from build123d import *

# Parameters (mm, degrees)
SKETCH1_R           = 82.5
BOSS_EXTRUDE1_DEPTH = 28
SKETCH2_R           = 10
CUT_EXTRUDE1_DEPTH  = 120.98541578
SKETCH3_R           = 7.474835821
CUT_EXTRUDE2_DEPTH  = 19.538331
CIRPATTERN1_START   = 8.461669322
CIRPATTERN1_DEPTH   = 19.538330678


# Read off the part's stored shape, not the designer's step: CirPattern1
with BuildPart() as part:
    # Sketch1 → Boss-Extrude1 (new body)
    with BuildSketch(Plane(origin=(0, 0, 0), x_dir=(1, 0, 0), z_dir=(0, 1, 0))):
        with Locations(Location((0, 0, 0), (0, 0, 270))):
            Circle(SKETCH1_R)
    extrude(amount=BOSS_EXTRUDE1_DEPTH)

    # Sketch2 → Cut-Extrude1 (cut, through all)
    with BuildSketch(Plane(origin=(0, 0, 0), x_dir=(1, 0, 0), z_dir=(0, 1, 0))):
        with Locations(Location((0, 0, 0), (0, 0, 270))):
            Circle(SKETCH2_R)
    extrude(amount=CUT_EXTRUDE1_DEPTH, mode=Mode.SUBTRACT)

    # Sketch3 → Cut-Extrude2 (cut)
    with BuildSketch(Plane(origin=(0, 28, 0), x_dir=(1, 0, 0), z_dir=(0, 1, 0))):
        with Locations((-17.151511033, 0)):
            Circle(SKETCH3_R)
    extrude(amount=-CUT_EXTRUDE2_DEPTH, mode=Mode.SUBTRACT)

    # CirPattern1 outline → CirPattern1 (cut)
    with BuildSketch(Plane(origin=(0, 0, 0), x_dir=(1, 0, 0), z_dir=(0, 1, 0)).offset(CIRPATTERN1_START)):
        with BuildLine():
            ThreePointArc((-1.654757081, 9.862138663), (0, 10), (1.654757081, 9.862138663))
            ThreePointArc((1.654757081, 9.862138663), (0, 24.626346854), (-1.654757081, 9.862138663))
        make_face()
        with BuildLine():
            ThreePointArc((9.862138663, -1.654757081), (24.626346854, 0), (9.862138663, 1.654757081))
            ThreePointArc((9.862138663, 1.654757081), (10, 0), (9.862138663, -1.654757081))
        make_face()
        with BuildLine():
            ThreePointArc((1.654757081, -9.862138663), (0, -10), (-1.654757081, -9.862138663))
            ThreePointArc((-1.654757081, -9.862138663), (0, -24.626346854), (1.654757081, -9.862138663))
        make_face()
    extrude(amount=CIRPATTERN1_DEPTH, mode=Mode.SUBTRACT)


solid = part.part
Read the model definition and answer for the solid it produces. Units are mm, in the model's axes. A direction names the side the tool comes from. Give positions to 0.01 mm unless a question says otherwise; leave off trailing zeros. Write each loop counter-clockwise with the first axis right and the second up, starting at its lowest first coordinate (ties: lowest second). Pieces come first, ordered by that corner, then holes. Notation, with made-up numbers: (-1, 37.5) - (6, 37.5) arc R22 cw to (6, 45.5) - close; hole circle Ø5 at (38.25, -14.75). An arc over 180 degrees is marked (long way). Answer in a Markdown table with one row per item. Add a question column.
Item 1: Section C-C, the plane z = 22 is taken. Write down the section's boundary in (x, y).
Item 2: Flat-ended cylindrical pins translate along their axes: P1, Ø1.5, axis at x = -16.5, y = 4, coming from the +Z side; P2, Ø1.5, axis at x = 45.5, y = 6, coming from the -Z side; P3, Ø4.5, axis at x = 18, z = 2, coming from the +Y side. Find the tip coordinate at first contact, or state that the pin passes through.
Item 3: Determine the mould class of faces 1 (the face through (-3.83, 13.804, 9.237)), 2 (the face through (1, 0, 17)), 3 (the face through (-80.54, 13.8, -17.88)) for opening direction X: pulls with the +X half, pulls with the -X half, needs draft (parallel to the pull), parting line crosses it, or undercut.
Item 4: A tool of negligible diameter and unlimited length cuts with its end or side. For faces 4 (the face through (24.62, 18.09, 0.31)), 5 (the face through (-17, 28, 17)), from which of +Z, -Z, +X, -X, +Y, -Y can it reach the whole face along a straight path? Write none if from no direction.
Item 5: Find the intervals of material crossed by L1, parallel to X at y = 20.5, z = 0; L2, parallel to X at y = 25.75, z = 2; L3, parallel to Z at x = 8, y = 24, in increasing order.
Item 6: Section B-B, the plane y = 24 is taken. Write down the section's boundary in (x, z).
Item 7: Section D-D, the plane x = -61 is taken. Write down the section's boundary in (y, z), and give its area (3 significant figures).
Item 8: Section A-A, the plane x = -5.5 is taken. Write down the section's boundary in (y, z), and give its area (3 significant figures).
Recorded:
| question | item | result |
|---|---|---|
| 1 | outline | (-79.51, 0) - (79.51, 0) - (79.51, 28) - (5.69, 28) - (5.69, 8.46) - (-5.69, 8.46) - (-5.69, 28) - (-79.51, 28) - close |
| 2 | P1 | stops at z = 80.98 |
| 2 | P2 | stops at z = -69.31 |
| 2 | P3 | stops at y = 8.46 |
| 3 | face 1 | undercut |
| 3 | face 2 | needs draft |
| 3 | face 3 | parting line crosses it |
| 4 | face 4 | +Y |
| 4 | face 5 | +Z, -Z, +X, -X, +Y |
| 5 | L1 | x = -82.5 to -24.63, 24.63 to 82.5 |
| 5 | L2 | x = -82.48 to -24.35, -9.95 to -9.8, 9.8 to 9.95, 24.35 to 82.48 |
| 5 | L3 | z = -82.11 to -6, 6 to 82.11 |
| 6 | outline | circle Ø165 at (0, 0); hole (-9.86, -1.65) arc R10 ccw to (-1.65, -9.86) arc R7.47 ccw (long way) to (1.65, -9.86) arc R10 ccw to (9.86, -1.65) arc R7.47 ccw (long way) to (9.86, 1.65) arc R10 ccw to (1.65, 9.86) arc R7.47 ccw (long way) to (-1.65, 9.86) arc R10 ccw to (-9.86, 1.65) arc R7.47 ccw (long way) to start |
| 7 | outline | (0, -55.55) - (28, -55.55) - (28, 55.55) - (0, 55.55) - close |
| 7 | area | 3,110 mm2 |
| 8 | outline | (0, -82.32) - (28, -82.32) - (28, -22.21) - (8.46, -22.21) - (8.46, -12.09) - (28, -12.09) - (28, -8.35) - (0, -8.35) - close; (0, 8.35) - (28, 8.35) - (28, 12.09) - (8.46, 12.09) - (8.46, 22.21) - (28, 22.21) - (28, 82.32) - (0, 82.32) - close |
| 8 | area | 3,750 mm2 |
